from build123d import *

# Parameters (mm, degrees)
SKETCH1_W            = 50.8
SKETCH1_H            = 38.1
EXTRUDE1_DEPTH       = 1.6002
SKETCH2_R            = 1.524
CUT_EXTRUDE1_DEPTH   = 1.6002
LPATTERN1_COUNT      = 2
LPATTERN1_PITCH      = 38.1
LPATTERN1_COUNT_DIR2 = 2
LPATTERN1_PITCH_DIR2 = 25.4


with BuildPart() as part:
    # Sketch1 → Extrude1 (new body)
    with BuildSketch(Plane.XY):
        with Locations((25.4, -19.05)):
            Rectangle(SKETCH1_W, SKETCH1_H)
    extrude(amount=EXTRUDE1_DEPTH)

    # Sketch2 → Cut-Extrude1 (cut)
    with BuildSketch(Plane.XY.offset(1.6002)):
        with Locations((6.35, -6.35)):
            Circle(SKETCH2_R)
    cut_extrude1 = extrude(amount=-CUT_EXTRUDE1_DEPTH, mode=Mode.SUBTRACT)

    # LPattern1: Cut-Extrude1 2 × 2
    with Locations(*[(i * LPATTERN1_PITCH, -j * LPATTERN1_PITCH_DIR2, 0) for i in range(LPATTERN1_COUNT) for j in range(LPATTERN1_COUNT_DIR2) if (i, j) != (0, 0)]):
        add(cut_extrude1, mode=Mode.SUBTRACT)


solid = part.part
Geometry check sheet. Reference: the model listing, model coordinates, mm. Give positions to 0.01 mm unless a question says otherwise; leave off trailing zeros. Order: outer loops, then holes, each group sorted by start corner. A loop starts at its lowest first (then second) coordinate and runs counter-clockwise, first axis right, second up.
1. Scan lines: line 1 (Y direction, x = 6.35, z = 0.65); line 2 (X direction, y = -5, z = 1.3). Record each from-to range of solid material in increasing order.
Completed:
line 1: y = -38.1 to -33.27, -30.23 to -7.87, -4.83 to 0
line 2: x = 0 to 5.64, 7.06 to 43.74, 45.16 to 50.8
2. Depth check by flat-ended pin: pin 1 (2.5 mm diameter, centred on x = 44.45, y = -31.75, fed in from +Z). Enter the tip coordinate at first touch or a pass-through.
Completed:
pin 1: passes through
3. Sectioned sample at C-C (x = 6.35). Record the boundary of the cut face in (y, z), then the cut area to 3 significant figures.
Completed:
outline: (-38.1, 0) - (-33.27, 0) - (-33.27, 1.6) - (-38.1, 1.6) - close; (-30.23, 0) - (-7.87, 0) - (-7.87, 1.6) - (-30.23, 1.6) - close; (-4.83, 0) - (0, 0) - (0, 1.6) - (-4.83, 1.6) - close
area: 51.2 mm2
4. Sectioned sample at B-B (z = 1). Record the boundary of the cut face in (x, y).
Completed:
outline: (0, -38.1) - (50.8, -38.1) - (50.8, 0) - (0, 0) - close; hole circle Ø3.05 at (6.35, -31.75); hole circle Ø3.05 at (6.35, -6.35); hole circle Ø3.05 at (44.45, -31.75); hole circle Ø3.05 at (44.45, -6.35)
5. Sectioned sample at A-A (y = -31.75). Record the boundary of the cut face in (x, z).
Completed:
outline: (0, 0) - (4.83, 0) - (4.83, 1.6) - (0, 1.6) - close; (7.87, 0) - (42.93, 0) - (42.93, 1.6) - (7.87, 1.6) - close; (45.97, 0) - (50.8, 0) - (50.8, 1.6) - (45.97, 1.6) - close
6. Draft check along Y on faces 1 (the face through (50.8, -19, 1)), 2 (the face through (6.15, -30.24, 0.81)), 3 (the face through (25, 0, 1)). Enter one of: pulls with the +Y half, pulls with the -Y half, needs draft (parallel to the pull), parting line crosses it, or undercut.
Completed:
face 1: needs draft
face 2: undercut
face 3: pulls with the +Y half
